from build123d import *

# Parameters (mm, degrees)
SKETCH1_R             = 12
SKETCH1_R_2           = 6
BOSS_EXTRUDE1_DEPTH   = 6
BOSS_EXTRUDE1_2_DEPTH = 6
BOSS_EXTRUDE2_DEPTH   = 3
BOSS_EXTRUDE3_DEPTH   = 9


with BuildPart() as part:
    # Sketch1 → Boss-Extrude1 (new, symmetric)
    with BuildSketch(Plane.XY):
        with Locations((-45, 0)):
            Circle(SKETCH1_R)
        with Locations((-45, 0)):
            Circle(SKETCH1_R_2, mode=Mode.SUBTRACT)
    extrude(amount=BOSS_EXTRUDE1_DEPTH, both=True)



with BuildPart() as body_2:
    # Sketch1 → Boss-Extrude1 2 (new, symmetric)
    with BuildSketch(Plane.XY):
        with Locations((45, 0)):
            Circle(SKETCH1_R)
        with Locations((45, 0)):
            Circle(SKETCH1_R_2, mode=Mode.SUBTRACT)
    extrude(amount=BOSS_EXTRUDE1_2_DEPTH, both=True)


with BuildPart() as part_1:
    add(part.part)

    add(body_2.part)  # Boss-Extrude2 merges body 2
    # Sketch3 → Boss-Extrude2 (add, symmetric)
    with BuildSketch(Plane.XY):
        with BuildLine():
            Line((-34.607695155, 6), (34.607695155, 6))
            ThreePointArc((34.607695155, 6), (33, 0), (34.607695155, -6))
            Line((34.607695155, -6), (-34.607695155, -6))
            ThreePointArc((-34.607695155, -6), (-33, 0), (-34.607695155, 6))
        make_face()
    extrude(amount=BOSS_EXTRUDE2_DEPTH, both=True)

    # Sketch4 → Boss-Extrude3 (add, symmetric)
    with BuildSketch(Plane.XY):
        with BuildLine():
            ThreePointArc((55.392304845, 6), (75.434547778, 9.446410386), (93.174330904, 19.389716726))
            ThreePointArc((93.174330904, 19.389716726), (98.763947455, 20.448721573), (102.725037233, 16.365209331))
            ThreePointArc((102.725037233, 16.365209331), (105, 0), (102.725037233, -16.365209331))
            ThreePointArc((102.725037233, -16.365209331), (98.763947455, -20.448721573), (93.174330904, -19.389716726))
            ThreePointArc((93.174330904, -19.389716726), (75.434547778, -9.446410386), (55.392304845, -6))
            ThreePointArc((55.392304845, -6), (57, 0), (55.392304845, 6))
        make_face()
    extrude(amount=BOSS_EXTRUDE3_DEPTH, both=True)


solid = part_1.part
Work out the finished part from the listing and answer in its coordinate system (mm). A direction names the side the tool comes from. Round coordinates to 2 decimals unless told otherwise and drop trailing zeros. Write each loop counter-clockwise with the first axis right and the second up, starting at its lowest first coordinate (ties: lowest second). Pieces come first, ordered by that corner, then holes.
1) A tool of negligible diameter and unlimited length cuts with its end or side. For faces 1 (the flat face through (-43, 6, -6)), 2 (the cylindrical face through (75.7, -9.54, 0.13)), 3 (the flat face through (0, 6, 0)), from which of +Z, -Z, +X, -X, +Y, -Y can it reach the whole face along a straight path? Write none if from no direction.
2) Straight lines are drawn through the part: line 1 (Y direction, x = -45, z = 3.75); line 2 (X direction, y = 5, z = -4); line 3 (X direction, y = -11, z = 2). For each, find the intervals that lie inside material, in ascending order.
3) Given pin 1 Ø7 at (x, y) = (-45, 0) entering from +Z; pin 2 Ø6 at (x, y) = (77, -12.5) entering from -Z; pin 3 Ø4 at (y, z) = (10, -1) entering from +X; pin 4 Ø19 at (x, y) = (-43.5, 2.5) entering from +Z, each flat-ended and moving along its own axis, determine where each tip first touches the part or whether it passes through.
4) The mould has two halves that part along Y. Classify faces 4 (the cylindrical face through (-56.99, 0.53, 0.08)), 5 (the flat face through (0, -6, 0)), 6 (the cylindrical face through (39, 0, 0)): pulls with the +Y half, pulls with the -Y half, needs draft (parallel to the pull), parting line crosses it, or undercut.
5) A cutting plane is placed at B-B (y = 0). Give the vertices of the cut face in (x, z), plus the area to 3 significant figures.
6) A cutting plane is placed at D-D (y = 9). Give the vertices of the cut face in (x, z).
7) A cutting plane is placed at C-C (z = 7.5). Give the vertices of the cut face in (x, y).
8) A cutting plane is placed at A-A (x = -45). Give the vertices of the cut face in (y, z), plus the area to 3 significant figures.
Completed:
1. face 1: -Z, -X, +Y, -Y
1. face 2: +Z, -Z, -Y
1. face 3: +Z, -Z, +Y
2. line 1: y = -12 to -6, 6 to 12
2. line 2: x = -55.91 to -48.32, -41.68 to -34.09, 34.09 to 41.68, 48.32 to 104.79
2. line 3: x = -49.8 to -40.2, 40.2 to 49.8, 79.37 to 103.98
3. pin 1: passes through
3. pin 2: stops at z = -9
3. pin 3: stops at x = 104.46
3. pin 4: stops at z = 6
4. face 4: parting line crosses it
4. face 5: pulls with the -Y half
4. face 6: undercut
5. outline: (-57, -6) - (-51, -6) - (-51, 6) - (-57, 6) - close; (-39, -6) - (-33, -6) - (-33, -3) - (33, -3) - (33, -6) - (39, -6) - (39, 6) - (33, 6) - (33, 3) - (-33, 3) - (-33, 6) - (-39, 6) - close; (51, -6) - (57, -6) - (57, -9) - (105, -9) - (105, 9) - (57, 9) - (57, 6) - (51, 6) - close
5. area: 1,550 mm2
6. outline: (-52.94, -6) - (-37.06, -6) - (-37.06, 6) - (-52.94, 6) - close; (37.06, -6) - (52.94, -6) - (52.94, 6) - (37.06, 6) - close; (74.13, -9) - (104.32, -9) - (104.32, 9) - (74.13, 9) - close
7. outline: (55.39, -6) arc R60 cw to (93.17, -19.39) arc R6 ccw to (102.73, -16.37) arc R60 ccw to (102.73, 16.37) arc R6 ccw to (93.17, 19.39) arc R60 cw to (55.39, 6) arc R12 cw to start
8. outline: (-12, -6) - (-6, -6) - (-6, 6) - (-12, 6) - close; (6, -6) - (12, -6) - (12, 6) - (6, 6) - close
8. area: 144 mm2
